Source: three-view drawing plus pictorial views. Frame: mm from the lowest corner of the part. Give positions to 0.01 mm unless a question says otherwise; leave off trailing zeros. Order: outer loops, then holes, each group sorted by start corner. A loop starts at its lowest first (then second) coordinate and runs counter-clockwise, first axis right, second up. Notation, with made-up numbers: M 38.25,24.5 L 80.25,24.5 A19 cw 80.25,45.5 Z; hole C 56,67 d8. An arc over 180 degrees is marked long. Use CSV: the item, a comma, the result in double quotes. Start each with the question number.
Item 1: Section query A-A on y = 20. Return loops of the section in (x, z), and give its area (3 significant figures).
Item 2: Ray query, probe 1 along Y at (x, z) = (46, 3); probe 2 along Y at (x, z) = (43, 3.8); probe 3 along X at (y, z) = (2, 0.8). Return the intervals inside material, ascending. Write a range as from..to.
Item 3: Section query D-D on y = 30. Return loops of the section in (x, z).
Item 4: Section query B-B on z = 2.7. Return loops of the section in (x, y).
Item 5: First-contact query: pin 1 (1.8 mm diameter, centred on x = 4, y = 20, fed in from +Z). Flat tip, straight axial feed; report the tip coordinate or a pass-through.
Item 6: Section query C-C on x = 4. Return loops of the section in (y, z).
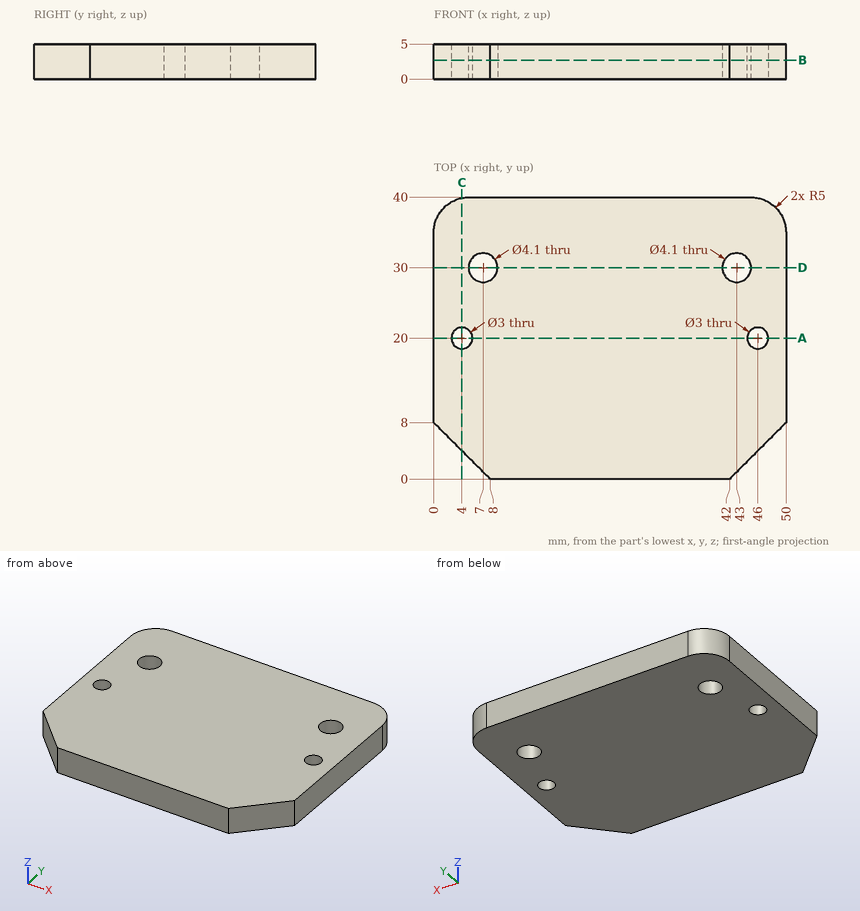
Verdict:
1,outline,"M 0,0 L 2.5,0 L 2.5,5 L 0,5 Z; M 5.5,0 L 44.5,0 L 44.5,5 L 5.5,5 Z; M 47.5,0 L 50,0 L 50,5 L 47.5,5 Z"
1,area,"220 mm2"
2,probe 1,"4..18.5, 21.5..39.9"
2,probe 2,"1..27.95, 32.05..40"
2,probe 3,"6..44"
3,outline,"M 0,0 L 4.95,0 L 4.95,5 L 0,5 Z; M 9.05,0 L 40.95,0 L 40.95,5 L 9.05,5 Z; M 45.05,0 L 50,0 L 50,5 L 45.05,5 Z"
4,outline,"M 0,8 L 8,0 L 42,0 L 50,8 L 50,35 A5 ccw 45,40 L 5,40 A5 ccw 0,35 Z; hole C 4,20 d3; hole C 7,30 d4.1; hole C 43,30 d4.1; hole C 46,20 d3"
5,pin 1,"through"
6,outline,"M 4,0 L 18.5,0 L 18.5,5 L 4,5 Z; M 21.5,0 L 39.9,0 L 39.9,5 L 21.5,5 Z"
